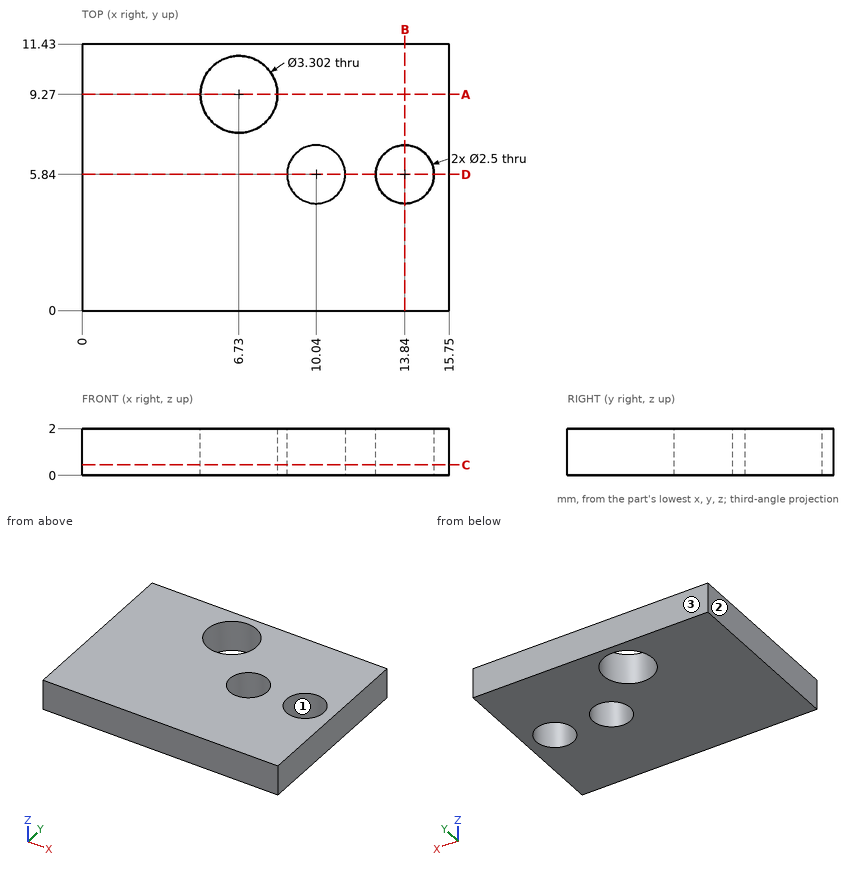
Source: three-view drawing plus pictorial views. Frame: mm from the lowest corner of the part. Coordinates: 2 decimals unless noted, no trailing zeros. Order: outer loops, then holes, each group sorted by start corner. A loop starts at its lowest first (then second) coordinate and runs counter-clockwise, first axis right, second up.
Item 1: Cut plane B-B (x = 13.84). Return loops of the section in (y, z), plus the area to 3 significant figures.
Output values:
outline: (0, 0) - (4.59, 0) - (4.59, 2) - (0, 2) - close; (7.09, 0) - (11.43, 0) - (11.43, 2) - (7.09, 2) - close
area: 17.9 mm2
Item 2: Cut plane A-A (y = 9.27). Return loops of the section in (x, z).
Output values:
outline: (0, 0) - (5.08, 0) - (5.08, 2) - (0, 2) - close; (8.38, 0) - (15.75, 0) - (15.75, 2) - (8.38, 2) - close
Item 3: Material intervals for line 1 (X direction, y = 9.27, z = 1.6); line 2 (Y direction, x = 6.73, z = 1.65); line 3 (X direction, y = 4.75, z = 0.5), sorted ascending.
Output values:
line 1: x = 0 to 5.08, 8.38 to 15.75
line 2: y = 0 to 7.62, 10.92 to 11.43
line 3: x = 0 to 9.43, 10.65 to 13.23, 14.45 to 15.75
Item 4: Pull-direction query (Y, two-part tool) for the marked faces 1, 2 and 3; classes: pulls with the +Y half, pulls with the -Y half, needs draft (parallel to the pull), parting line crosses it, or undercut.
Output values:
face 1: undercut
face 2: needs draft
face 3: pulls with the +Y half
Item 5: Cut plane D-D (y = 5.84). Return loops of the section in (x, z).
Output values:
outline: (0, 0) - (8.79, 0) - (8.79, 2) - (0, 2) - close; (11.29, 0) - (12.59, 0) - (12.59, 2) - (11.29, 2) - close; (15.09, 0) - (15.75, 0) - (15.75, 2) - (15.09, 2) - close
Item 6: Cut plane C-C (z = 0.45). Return loops of the section in (x, y), plus the area to 3 significant figures.
Output values:
outline: (0, 0) - (15.75, 0) - (15.75, 11.43) - (0, 11.43) - close; hole circle Ø3.3 at (6.73, 9.27); hole circle Ø2.5 at (10.04, 5.84); hole circle Ø2.5 at (13.84, 5.84)
area: 162 mm2
